```python
from build123d import *

# Parameters (mm, degrees)
F1_DEPTH = 10
F2_R     = 1
F3_R     = 0.6
F4_DEPTH = 2.5


with BuildPart() as f1:
    # F0 (on Front) → F1 (new body)
    with BuildSketch(Plane.XZ):
        with BuildLine():
            Line((7.5, 55.5), (10, 55.5))
            ThreePointArc((10, 55.5), (0, 65.5), (-10, 55.5))
            Line((-10, 55.5), (-7.5, 55.5))
            ThreePointArc((-7.5, 55.5), (0, 63), (7.5, 55.5))
        make_face()
    extrude(amount=F1_DEPTH)

    # F2
    f2_edges = [f1.edges().sort_by_distance(p)[0] for p in [
        (0, 0, 65.5),
        (0, -10, 65.5),
    ]]
    fillet(f2_edges, radius=F2_R)

    # F3 (on face) → F4 (cut)
    with BuildSketch(Plane(origin=(0, 0, 55.5), x_dir=(1, 0, 0), z_dir=(0, 0, -1))):
        with Locations((8.75, 1.5)):
            Circle(F3_R)
        with Locations((8.75, 8.5)):
            Circle(F3_R)
        with Locations((-8.75, 1.5)):
            Circle(F3_R)
        with Locations((-8.75, 8.5)):
            Circle(F3_R)
    extrude(amount=-F4_DEPTH, mode=Mode.SUBTRACT)


solid = f1.part
```
The listing builds one solid part. Answer for the finished solid, in the listing's coordinates (mm). A direction names the side the tool comes from. Coordinates: 2 decimals unless noted, no trailing zeros. Write each loop counter-clockwise with the first axis right and the second up, starting at its lowest first coordinate (ties: lowest second). Pieces come first, ordered by that corner, then holes. Notation, with made-up numbers: (-0.5, -16.5) - (10.5, -16.5) arc R17 cw to (10.5, 16.5) - close; hole circle Ø2 at (27.5, -26). An arc over 180 degrees is marked (long way). Return JSON: item names as keys, results as strings. Group by question number.
1. Which of the six approach directions +Z, -Z, +X, -X, +Y, -Y give full straight-line access (tool end or side, diameter ignored) to faces 4 (the flat face through (-8.8, -8.5, 58)), 5 (the flat face through (-9, -5, 55.5))?
2. A cutting plane is placed at C-C, the plane y = -4. Determine the outline of the cut face in (x, z).
3. A cutting plane is placed at B-B, the plane y = -1.5. Determine the outline of the cut face in (x, z).
4. Determine the mould class of faces 1 (the flat face through (8.7, -1.5, 58)), 2 (the cylindrical face through (0.2, -4.9, 65.5)), 3 (the flat face through (0, 0, 63.4)) for opening direction X: released by +X, released by -X, zero draft, split by the parting line, or undercut.
5. Given pin 1 (5 mm diameter, centred on x = 2, y = -6, fed in from +Z); pin 2 (1.1 mm diameter, centred on x = 8.75, y = -8.5, fed in from -Z); pin 3 (1 mm diameter, centred on x = 5.5, z = 58.5, fed in from -Y); pin 4 (5 mm diameter, centred on x = 3.5, y = -8, fed in from +Z), each flat-ended and moving along its own axis, determine where each tip first touches the part or whether it passes through.
6. Straight lines are drawn through the part: L1, parallel to Y at x = -8.75, z = 56.1; L2, parallel to X at y = -1.5, z = 56.5; L3, parallel to X at y = -8.5, z = 56.3. For each, find the intervals that lie inside material, in ascending order.
7. A cutting plane is placed at D-D, the plane y = -0.25. Determine the outline of the cut face in (x, z), plus the area to 3 significant figures.
8. A cutting plane is placed at A-A, the plane x = 0. Determine the outline of the cut face in (y, z), plus the area to 3 significant figures.
Ans:
{
 "1": {"face 4": "-Z", "face 5": "-Z, +X, -X, +Y, -Y"},
 "2": {"outline": "(-10, 55.5) - (-7.5, 55.5) arc R7.5 cw to (7.5, 55.5) - (10, 55.5) arc R10 ccw to start"},
 "3": {"outline": "(-10, 55.5) - (-9.35, 55.5) - (-9.35, 58) - (-8.15, 58) - (-8.15, 55.5) - (-7.5, 55.5) arc R7.5 cw to (7.5, 55.5) - (8.15, 55.5) - (8.15, 58) - (9.35, 58) - (9.35, 55.5) - (10, 55.5) arc R10 ccw to start"},
 "4": {"face 1": "undercut", "face 2": "split by the parting line", "face 3": "zero draft"},
 "5": {"pin 1": "z = 65.5", "pin 2": "z = 58", "pin 3": "through", "pin 4": "z = 65.45"},
 "6": {"L1": "-10 to -9.1, -7.9 to -2.1, -0.9 to 0", "L2": "-9.95 to -9.35, -8.15 to -7.43, 7.43 to 8.15, 9.35 to 9.95", "L3": "-9.97 to -9.35, -8.15 to -7.46, 7.46 to 8.15, 9.35 to 9.97"},
 "7": {"outline": "(-9.66, 55.5) - (-7.5, 55.5) arc R7.5 cw to (7.5, 55.5) - (9.66, 55.5) arc R9.66 ccw to start", "area": "58.3 mm²"},
 "8": {"outline": "(-10, 63) - (0, 63) - (0, 64.5) arc R1 ccw to (-1, 65.5) - (-9, 65.5) arc R1 ccw to (-10, 64.5) - close", "area": "24.6 mm²"}
}
